Autodesk Inventor part; units mm, degrees
ref_plane "YZ Plane" through (0, 0, 0) normal (1, 0, 0) x (0, 1, 0)
ref_plane "XZ Plane" through (0, 0, 0) normal (0, 1, 0) x (-1, 0, 0)
ref_plane "XY Plane" through (0, 0, 0) normal (0, 0, 1) x (1, 0, 0)
sketch "Sketch1" plane through (0, 0, 0) normal (0, 1, 0) x (-1, 0, 0)
  arc A0 (-63, 48) -> (-63, -48) centre (-63, 0) ccw
  line L0 (0, -30.052) -> (0, -21.9885) construction
  circle A1 centre (-63, 0) radius 37.5
  circle A2 centre (-63, 0) radius 42 construction
  line L1 (-63, -48) -> (0, -48)
  line L2 (-63, 48) -> (0, 48)
  line L3 (0, 0) -> (-63, 0) construction
  circle A3 centre (-63, -42) radius 2
  circle A4 centre (-33.3015, -29.6985) radius 2
  circle A5 centre (-21, 0) radius 2
  circle A6 centre (-33.3015, 29.6985) radius 2
  circle A7 centre (-63, 42) radius 2
  circle A8 centre (-92.6985, 29.6985) radius 2
  circle A9 centre (-105, 0) radius 2
  circle A10 centre (-92.6985, -29.6985) radius 2
  arc A11 (63, -48) -> (63, 48) centre (63, 0) ccw
  circle A12 centre (63, 0) radius 37.5
  circle A13 centre (63, 0) radius 42 construction
  line L4 (63, -48) -> (0, -48)
  line L5 (63, 48) -> (0, 48)
  line L6 (0, 0) -> (63, 0) construction
  circle A14 centre (63, -42) radius 2
  circle A15 centre (33.3015, -29.6985) radius 2
  circle A16 centre (21, 0) radius 2
  circle A17 centre (33.3015, 29.6985) radius 2
  circle A18 centre (63, 42) radius 2
  circle A19 centre (92.6985, 29.6985) radius 2
  circle A20 centre (105, 0) radius 2
  circle A21 centre (92.6985, -29.6985) radius 2
  line L7 (0, 0) -> (0, -5) construction
  circle A22 centre (0, -5) radius 2
  line L8 (0, 0) -> (0, 5)
  circle A23 centre (0, 5) radius 2
  line L9 (0, -48) -> (0, -40) construction
  circle A24 centre (0, -40) radius 2
  line L10 (0, -40) -> (0, -30) construction
  circle A25 centre (0, -30) radius 2
  line L11 (0, 30.052) -> (0, 21.9885) construction
  line L12 (0, 48) -> (0, 40) construction
  circle A26 centre (0, 40) radius 2
  line L13 (0, 40) -> (0, 30) construction
  circle A27 centre (0, 30) radius 2
  dimension "d4" = 84
  dimension "d2" = 96
  dimension "d3" = 75
  dimension "d5" = 63
  dimension "d6" = 4
  dimension "d9" = 360
  dimension "d24" = 5
  dimension "d25" = 4
  dimension "d26" = 5
  dimension "d27" = 4
  dimension "d32" = 8
  dimension "d33" = 4
  dimension "d34" = 10
  dimension "d35" = 4
extrude "Extrusion1" add sketch "Sketch1" along normal blind 3
chamfer "Chamfer1" distance 2 angle 45 16 edges at (-19, 3, 0) (-31.3015, 3, -29.6985) (-61, 3, -42) (-90.6985, 3, -29.6985) (-103, 3, 0) (-90.6985, 3, 29.6985) (-61, 3, 42) (-31.3015, 3, 29.6985) (35.3015, 3, 29.6985) (23, 3, 0) (35.3015, 3, -29.6985) (65, 3, -42) (94.6985, 3, -29.6985) (107, 3, 0) (94.6985, 3, 29.6985) (65, 3, 42)
properties part number "leg_connector"
For this review, take the finished solid that the model builds, in its own axes (mm). Give positions to 0.01 mm unless a question says otherwise; leave off trailing zeros. Write each loop counter-clockwise with the first axis right and the second up, starting at its lowest first coordinate (ties: lowest second). Pieces come first, ordered by that corner, then holes. Notation, with made-up numbers: M -23.75,39.5 L -18.75,39.5 A32 cw -18.75,69.5 Z; hole C 46.25,76.25 d4. An arc over 180 degrees is marked long. One line per item, written item: value.
1) The part is to be moulded in two halves that separate along Z. For faces 1 (the conical face through (-61.43, 1.13, 43.44)), 2 (the conical face through (-102.877, 1.125, 0.093)), say which applies: +Z half, -Z half, draft (parallel to the pull), parting line (faces both ways), or undercut.
Results are:
face 1: undercut
face 2: undercut
2) For P1, Ø5, axis at x = -33.3, z = 29.7, coming from the +Y side; P2, Ø6.5, axis at x = -92.7, z = 29.7, coming from the +Y side, all flat-tipped, find the tip position at first contact; note any pin that passes through.
Results are:
P1: stops at y = 1.5
P2: stops at y = 2.25
3) For line 1 (Z direction, x = -31.5, y = 0.3); line 2 (Z direction, x = 63, y = 0.8); line 3 (X direction, y = 1.4, z = 41.5), list the stretches that pass through material, from the lowest coordinate up. Write a range as from..to.
Results are:
line 1: z = -48..-30.57, -28.83..-20.35, 20.35..28.83, 30.57..48
line 2: z = -48..-44, -40..-37.5, 37.5..40, 44..48
line 3: x = -87.12..-65.35, -60.65..-1.32, 1.32..60.65, 65.35..87.12
4) Take a section at A-A, the plane x = -21. Write out the cut boundary in (y, z), then the cut area to 3 significant figures.
Results are:
outline: M 0,-48 L 3,-48 L 3,-4 L 1,-2 L 0,-2 Z; M 0,2 L 1,2 L 3,4 L 3,48 L 0,48 Z
area: 272 mm²
5) Take a section at B-B, the plane z = 0. Count the separate pieces of the cut face and the enclosed holes in it, then the cut area to 3 significant figures.
Results are:
separate pieces: 7
enclosed holes: 0
area: 152 mm²
6) Take a section at D-D, the plane x = -105. Write out the cut boundary in (y, z), then the cut area to 3 significant figures.
Results are:
outline: M 0,-23.24 L 3,-23.24 L 3,-4 L 1,-2 L 0,-2 Z; M 0,2 L 1,2 L 3,4 L 3,23.24 L 0,23.24 Z
area: 123 mm²
